For this review, use the dimensioned drawing (mm, ordinates from the lowest corner) and the shaded views. A direction names the side the tool comes from. Coordinates: 2 decimals unless noted, no trailing zeros. Order: outer loops, then holes, each group sorted by start corner. A loop starts at its lowest first (then second) coordinate and runs counter-clockwise, first axis right, second up. Notation, with made-up numbers: M 57.5,-22 L 76.5,-22 A36 cw 76.5,12 Z; hole C 32.25,-18 d6. An arc over 180 degrees is marked long. Write each question's results on one line, items separated by ' | '.
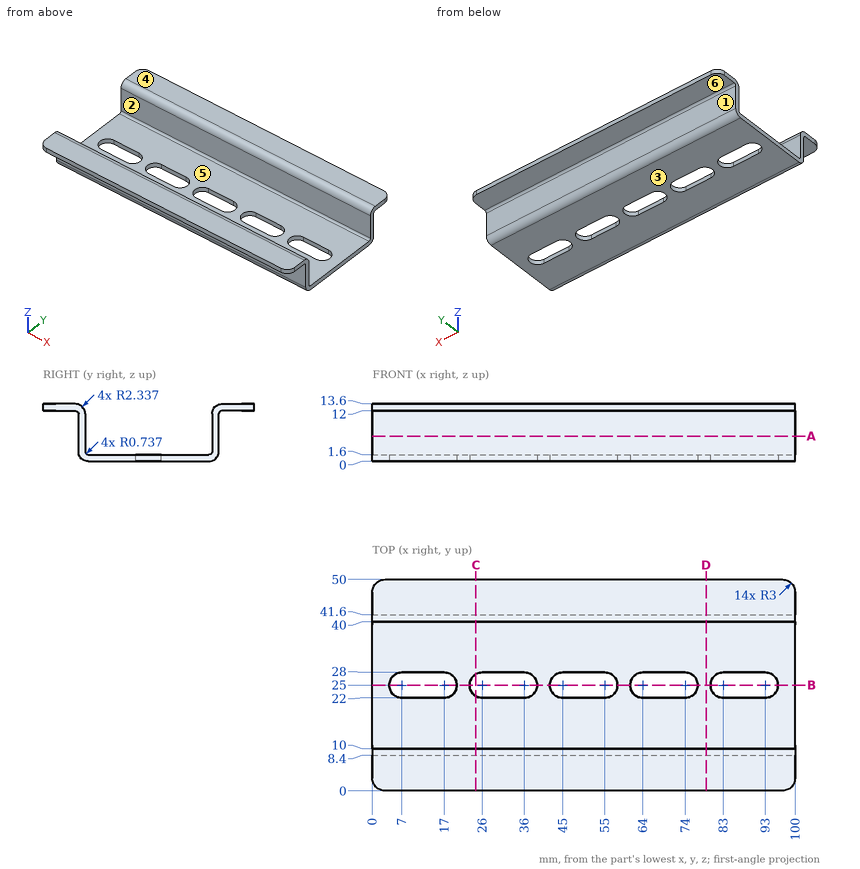
1) To check wall thickness, follow line 1 along Y through (x, z) = (17.5, 5.5); line 2 along Z through (x, y) = (21.5, 23); line 3 along Y through (x, z) = (56, 13) (1 decimal). State the ranges of each line that lie inside material, in increasing order.
Solutions:
line 1: 8.4 to 10, 40 to 41.6 | line 2: 0 to 1.6 | line 3: 0 to 9.2, 40.8 to 50
2) Take a section at D-D on x = 79. State the section outline as (y, z) points, plus the area to 3 significant figures.
Solutions:
outline: M 0,12 L 7.66,12 A0.74 cw 8.4,11.26 L 8.4,2.34 A2.34 ccw 10.74,0 L 39.26,0 A2.34 ccw 41.6,2.34 L 41.6,11.26 A0.74 cw 42.34,12 L 50,12 L 50,13.6 L 42.34,13.6 A2.34 ccw 40,11.26 L 40,2.34 A0.74 cw 39.26,1.6 L 10.74,1.6 A0.74 cw 10,2.34 L 10,11.26 A2.34 ccw 7.66,13.6 L 0,13.6 Z | area: 114 mm2
3) The part is to be moulded in two halves that separate along Y. For the marked faces 1, 2 and 3, say which applies: pulls with the +Y half, pulls with the -Y half, needs draft (parallel to the pull), parting line crosses it, or undercut.
Solutions:
face 1: pulls with the +Y half | face 2: undercut | face 3: needs draft
4) Take a section at A-A on z = 6. State the section outline as (x, y) points.
Solutions:
outline: M 0,8.4 L 100,8.4 L 100,10 L 0,10 Z; M 0,40 L 100,40 L 100,41.6 L 0,41.6 Z
5) Take a section at B-B on y = 25. State the section outline as (x, z) points.
Solutions:
outline: M 0,0 L 4,0 L 4,1.6 L 0,1.6 Z; M 20,0 L 23,0 L 23,1.6 L 20,1.6 Z; M 39,0 L 42,0 L 42,1.6 L 39,1.6 Z; M 58,0 L 61,0 L 61,1.6 L 58,1.6 Z; M 77,0 L 80,0 L 80,1.6 L 77,1.6 Z; M 96,0 L 100,0 L 100,1.6 L 96,1.6 Z
6) Take a section at C-C on x = 24.5. State the section outline as (y, z) points, plus the area to 3 significant figures.
Solutions:
outline: M 0,12 L 7.66,12 A0.74 cw 8.4,11.26 L 8.4,2.34 A2.34 ccw 10.74,0 L 22.4,0 L 22.4,1.6 L 10.74,1.6 A0.74 cw 10,2.34 L 10,11.26 A2.34 ccw 7.66,13.6 L 0,13.6 Z; M 27.6,0 L 39.26,0 A2.34 ccw 41.6,2.34 L 41.6,11.26 A0.74 cw 42.34,12 L 50,12 L 50,13.6 L 42.34,13.6 A2.34 ccw 40,11.26 L 40,2.34 A0.74 cw 39.26,1.6 L 27.6,1.6 Z | area: 106 mm2
7) For the marked faces 4, 5 and 6, list the 3-axis set-ups (+Z, -Z, +X, -X, +Y, -Y) from which the entire face can be reached by the end or side of a thin tool; tool diameter is ignored.
Solutions:
face 4: +Z, +X, -X, +Y, -Y | face 5: +Z, +X, -X | face 6: -Z, +X, -X, +Y
8) For pin 1 (5 mm diameter, centred on x = 12, z = 10.5, fed in from +Y); pin 2 (1.8 mm diameter, centred on x = 88.5, z = 1, fed in from -Y); pin 3 (1.5 mm diameter, centred on x = 87, z = 4.5, fed in from +Y); pin 4 (0.8 mm diameter, centred on x = 14.5, z = 1, fed in from -Y) (1 decimal), all flat-tipped, find the tip position at first contact; note any pin that passes through.
Solutions:
pin 1: y = 50 | pin 2: y = 8.44 | pin 3: y = 41.6 | pin 4: y = 8.6
